from build123d import *

# Parameters (mm, degrees)
F1_DEPTH  = 20
F2_DEPTH  = 15
F3_W      = 8
F3_H      = 0.1715728753
F4_DEPTH  = 35.001
F6_DEPTH  = 15
F7_SIZE   = 1.24999
F8_DEPTH  = 7.9
F9_W      = 8
F9_H      = 6.8284271247
F10_DEPTH = 3
F13_DEPTH = 3
F15_DEPTH = 8.001
F17_DEPTH = 60.901
F19_DEPTH = 8.001
F20_SIZE  = 1
F21_SIZE  = 0.5


# Not quite as in the source:
# - a fillet or chamfer is up to 0.001 mm smaller than in the source, because OpenCascade refuses the exact size


with BuildPart() as f1:
    # F0 (on Top) → F1 (new body)
    with BuildSketch(Plane.XY):
        with BuildLine():
            ThreePointArc((-1, -2.8284271247), (0, 3), (1, -2.8284271247))
            Line((1, -2.8284271247), (1, -3))
            Line((1, -3), (4, -3))
            Line((4, -3), (4, 4))
            Line((4, 4), (0, 4))
            Line((0, 4), (-4, 4))
            Line((-4, 4), (-4, -3))
            Line((-4, -3), (-1, -3))
            Line((-1, -3), (-1, -2.8284271247))
        make_face()
    extrude(amount=F1_DEPTH)

    # F2 (add): a face of the model
    f2_faces = [f1.faces().sort_by_distance(p)[0] for p in [
        (0, 3.1063014581, 20),
    ]]
    extrude(f2_faces, amount=F2_DEPTH)

    # F3 (on face) → F4 (cut, through all)
    with BuildSketch(Plane.XY.offset(35)):
        with Locations((0, -2.9142135624)):
            Rectangle(F3_W, F3_H)
    extrude(amount=-F4_DEPTH, mode=Mode.SUBTRACT)

    # F5 (on face) → F6 (join)
    with BuildSketch(Plane.XY.offset(35)):
        with BuildLine():
            ThreePointArc((-1, -1.4361406616), (0, 1.75), (1, -1.4361406616))
            Line((1, -1.4361406616), (0.25, -2.1322838932))
            Line((0.25, -2.1322838932), (1, -2.8284271247))
            Line((1, -2.8284271247), (4, -2.8284271247))
            Line((4, -2.8284271247), (4, 4))
            Line((4, 4), (-4, 4))
            Line((-4, 4), (-4, -2.8284271247))
            Line((-4, -2.8284271247), (-1, -2.8284271247))
            Line((-1, -2.8284271247), (-0.25, -2.1322838932))
            Line((-0.25, -2.1322838932), (-1, -1.4361406616))
        make_face()
    extrude(amount=F6_DEPTH)

    # F7 (size 1.25 in the source; OpenCascade refuses exactly that, so slightly less here)
    f7_edges = [f1.edges().sort_by_distance(p)[0] for p in [
        (0, 1.75, 35),
    ]]
    chamfer(f7_edges, length=F7_SIZE)

    # F8 (add): a face of the model
    f8_faces = [f1.faces().sort_by_distance(p)[0] for p in [
        (-2.5, -2.7232475559, 0),
    ]]
    extrude(f8_faces, amount=F8_DEPTH)

    # F9 (on face) → F10 (join)
    with BuildSketch(Plane(origin=(0, 0, -7.9), x_dir=(1, 0, 0), z_dir=(0, 0, -1))):
        with Locations((0, -0.5857864376)):
            Rectangle(F9_W, F9_H)
    extrude(amount=F10_DEPTH)

    # F12 (on face) → F13 (cut)
    with BuildSketch(Plane.XZ.offset(2.8284271247)):
        Polygon((0, 3.2961524227), (-3, -7.9), (1, -7.9), (3, -7.9), align=None)
    extrude(amount=-F13_DEPTH, mode=Mode.SUBTRACT)

    # F14 (on face) → F15 (cut, through all)
    with BuildSketch(Plane(origin=(-4, 0, 0), x_dir=(0, -1, 0), z_dir=(-1, 0, 0))):
        Polygon((-4, 46.0576057614), (2.8284271247, 50), (-4, 50), align=None)
    extrude(amount=-F15_DEPTH, mode=Mode.SUBTRACT)

    # F16 (on face) → F17 (cut, through all)
    with BuildSketch(Plane(origin=(0, 0, -10.9), x_dir=(1, 0, 0), z_dir=(0, 0, -1))):
        Polygon((4, -0.8309159426), (2.1703284663, -4), (4, -4), align=None)
        Polygon((-2.1703284663, -4), (-4, -0.8309159426), (-4, -4), align=None)
    extrude(amount=-F17_DEPTH, mode=Mode.SUBTRACT)

    # F18 (on face) → F19 (cut, through all)
    with BuildSketch(Plane.YZ.offset(4)):
        Polygon((4, 1.6660254038), (-2.8284271247, -2.2763688348), (-2.8284271247, -10.9), (4, -10.9), align=None)
    extrude(amount=-F19_DEPTH, mode=Mode.SUBTRACT)

    # F20
    f20_edges = [f1.edges().sort_by_distance(p)[0] for p in [
        (-4, -2.828427, 23.861816),
        (4, -2.828427, 23.861816),
    ]]
    chamfer(f20_edges, length=F20_SIZE)

    # F21
    f21_edges = [f1.edges().sort_by_distance(p)[0] for p in [
        (-2.170328, 4, 23.861816),
        (0, 4, 46.057606),
        (2.170328, 4, 23.861816),
        (0, 4, 1.666025),
    ]]
    chamfer(f21_edges, length=F21_SIZE)


solid = f1.part
Design review of the part built by this model. Coordinates are the model's own, in mm. A direction names the side the tool comes from. Coordinates: 2 decimals unless noted, no trailing zeros. Order: outer loops, then holes, each group sorted by start corner. A loop starts at its lowest first (then second) coordinate and runs counter-clockwise, first axis right, second up. Notation, with made-up numbers: (45.25, 70) - (49.25, 70) arc R22 ccw to (49.25, 87) - close; hole circle Ø7 at (-15.75, 75). An arc over 180 degrees is marked (long way). Put each result on its own line as item: value.
1) Wall thickness on L1, parallel to X at y = 0, z = 41.5; L2, parallel to X at y = 0, z = 15; L3, parallel to Y at x = -0.25, z = 31: over which ranges is each line inside the solid? List them lowest first. Write a range as from..to.
Response values:
L1: x = -4..-1.75, 1.75..4
L2: x = -4..-3, 3..4
L3: y = 2.99..4
2) The part is to be moulded in two halves that separate along X. For faces 3 (the face through (0, 2, 36)), 4 (the face through (-4, 0, 24)), 5 (the face through (-0.945, 1.835, 47.307)), say which applies: released by +X, released by -X, zero draft, split by the parting line, or undercut.
Response values:
face 3: undercut
face 4: released by -X
face 5: zero draft
3) Take a section at B-B, the plane x = -3.5. Give the boundary of the cut face in (y, z), and give its area (3 significant figures).
Response values:
outline: (-2.33, -1.99) - (1.7, 0.34) - (1.7, 47.39) - (-2.33, 49.71) - close
area: 199 mm²
4) Take a section at A-A, the plane z = 27.5. Give the boundary of the cut face in (x, y).
Response values:
outline: (-4, -1.83) - (-3, -2.83) - (-1, -2.83) arc R3 cw (long way) to (1, -2.83) - (3, -2.83) - (4, -1.83) - (4, 0.83) - (2.42, 3.57) - (1.67, 4) - (-1.67, 4) - (-2.42, 3.57) - (-4, 0.83) - close
5) Tool access review of faces 1 (the face through (0, 3, 17)), 2 (the face through (-2, -2.828, 24)): name each direction out of +Z, -Z, +X, -X, +Y, -Y from which nothing blocks a thin tool from reaching the whole face with its end or side.
Response values:
face 1: -Z
face 2: +Z, -Z, +X, -X, -Y
